```python
from build123d import *

# Parameters (mm, degrees)
SKETCH007_R           = 2.1
PAD004_DEPTH          = 1.83
CHAMFER_SIZE          = 1.6
SKETCH010_R           = 6
SKETCH010_W           = 10.4
SKETCH010_H           = 8.5
POCKET003_DEPTH       = 5
SKETCH012_R           = 3
SKETCH012_R_2         = 1.45
PAD005_DEPTH          = 4.5
SKETCH011_R           = 1.75
SKETCH011_R_2         = 3.5
SKETCH011_W           = 60.65
SKETCH011_H           = 46.16
POCKET004_DEPTH       = 7.5
CHAMFER001_SIZE       = 1
SKETCH013_W           = 70.5
SKETCH013_H           = 53
POCKET005_DEPTH       = 5
POCKET005_FACE89_R    = 1.45
PAD006_DEPTH          = 0.001
PAD006_FACE88_W       = 4.5
PAD006_FACE88_H       = 3.73839
PAD007_DEPTH          = 0.001
SKETCH014_W           = 13
SKETCH014_H           = 2.5
SKETCH014_W_2         = 8
PAD008_DEPTH          = 17
SKETCH015_R           = 1.6
POCKET006_DEPTH       = 16
PAD009_DEPTH          = 1.83
SKETCH017_R           = 1.625
POCKET007_DEPTH       = 5
SKETCH018_R           = 3
PAD010_DEPTH          = 1
SKETCH019_W           = 20
SKETCH019_H           = 10
POCKET008_DEPTH       = 1.831
POCKET008_DEPTH_BACK  = 17.001
POCKET008_FACE112_R   = 3
POCKET008_FACE112_R_2 = 1.45
PAD011_DEPTH          = 12.5
PAD011_FACE77_R       = 1.45
PAD012_DEPTH          = 12.5


with BuildPart() as part:
    # Sketch007 → Pad004 (new body)
    with BuildSketch(Plane.YZ):
        with BuildLine():
            ThreePointArc((185, 49.2), (183.857716, 51.957716), (181.1, 53.1))
            Line((-2.1, 53.1), (181.1, 53.1))
            ThreePointArc((-2.1, 53.1), (-4.857716, 51.957716), (-6, 49.2))
            Line((-6, -9), (-6, 49.2))
            ThreePointArc((-6, -9), (-4.857716, -11.757716), (-2.1, -12.9))
            Line((181.1, -12.9), (-2.1, -12.9))
            ThreePointArc((181.1, -12.9), (183.857716, -11.757716), (185, -9))
            Line((185, 49.2), (185, -9))
        make_face()
        with Locations((180.25, 49.11)):
            Circle(SKETCH007_R, mode=Mode.SUBTRACT)
        with Locations((180.25, -8.91)):
            Circle(SKETCH007_R, mode=Mode.SUBTRACT)
        with Locations((-1.25, -8.91)):
            Circle(SKETCH007_R, mode=Mode.SUBTRACT)
        with Locations((-1.25, 49.11)):
            Circle(SKETCH007_R, mode=Mode.SUBTRACT)
    extrude(amount=-PAD004_DEPTH)

    # Chamfer
    chamfer_edges = [part.edges().sort_by_distance(p)[0] for p in [
        (-1.83, 178.15, -8.91),
        (-1.83, 178.15, 49.11),
        (-1.83, -3.35, 49.11),
        (-1.83, -3.35, -8.91),
    ]]
    chamfer(chamfer_edges, length=CHAMFER_SIZE)

    # Sketch010 → Pocket003 (cut)
    with BuildSketch(Plane.YZ):
        with Locations((121.17, 7)):
            Circle(SKETCH010_R)
        with Locations((102.17, 7)):
            Circle(SKETCH010_R)
        with Locations((133.08, 5.25)):
            Rectangle(SKETCH010_W, SKETCH010_H)
        with BuildLine():
            ThreePointArc((174.5, 47.45), (172, 49.95), (169.5, 47.45))
            Line((169.5, 47.45), (169.5, -7.55))
            ThreePointArc((169.5, -7.55), (172, -10.05), (174.5, -7.55))
            Line((174.5, -7.55), (174.5, 47.45))
        make_face()
        with BuildLine():
            ThreePointArc((168.5, 47.45), (166, 49.95), (163.5, 47.45))
            Line((163.5, 47.45), (163.5, -7.55))
            ThreePointArc((163.5, -7.55), (166, -10.05), (168.5, -7.55))
            Line((168.5, -7.55), (168.5, 47.45))
        make_face()
        with BuildLine():
            ThreePointArc((162.5, 47.45), (160, 49.95), (157.5, 47.45))
            Line((157.5, 47.45), (157.5, -7.55))
            ThreePointArc((157.5, -7.55), (160, -10.05), (162.5, -7.55))
            Line((162.5, -7.55), (162.5, 47.45))
        make_face()
        with BuildLine():
            ThreePointArc((156.5, 47.45), (154, 49.95), (151.5, 47.45))
            Line((151.5, 47.45), (151.5, -7.55))
            ThreePointArc((151.5, -7.55), (154, -10.05), (156.5, -7.55))
            Line((156.5, -7.55), (156.5, 47.45))
        make_face()
        with BuildLine():
            ThreePointArc((150.5, 47.45), (148, 49.95), (145.5, 47.45))
            Line((145.5, 47.45), (145.5, -7.55))
            ThreePointArc((145.5, -7.55), (148, -10.05), (150.5, -7.55))
            Line((150.5, -7.55), (150.5, 47.45))
        make_face()
        with BuildLine():
            ThreePointArc((144.5, 47.45), (142, 49.95), (139.5, 47.45))
            Line((139.5, 47.45), (139.5, -7.55))
            ThreePointArc((139.5, -7.55), (142, -10.05), (144.5, -7.55))
            Line((144.5, -7.55), (144.5, 47.45))
        make_face()
    extrude(amount=-POCKET003_DEPTH, mode=Mode.SUBTRACT)

    # Sketch012 → Pad005 (join)
    with BuildSketch(Plane.YZ):
        with Locations((3.90349, -3.209935)):
            Circle(SKETCH012_R)
        with Locations((3.90349, -3.209935)):
            Circle(SKETCH012_R_2, mode=Mode.SUBTRACT)
        with Locations((3.90349, 41.790065)):
            Circle(SKETCH012_R)
        with Locations((3.90349, 41.790065)):
            Circle(SKETCH012_R_2, mode=Mode.SUBTRACT)
        with Locations((78.90349, 41.790065)):
            Circle(SKETCH012_R)
        with Locations((78.90349, 41.790065)):
            Circle(SKETCH012_R_2, mode=Mode.SUBTRACT)
        with Locations((120.90349, 41.790065)):
            Circle(SKETCH012_R)
        with Locations((120.90349, 41.790065)):
            Circle(SKETCH012_R_2, mode=Mode.SUBTRACT)
        with Locations((120.90349, 26.790065)):
            Circle(SKETCH012_R)
        with Locations((120.90349, 26.790065)):
            Circle(SKETCH012_R_2, mode=Mode.SUBTRACT)
        with Locations((78.90349, -3.209935)):
            Circle(SKETCH012_R)
        with Locations((78.90349, -3.209935)):
            Circle(SKETCH012_R_2, mode=Mode.SUBTRACT)
    extrude(amount=PAD005_DEPTH)

    # Sketch011 → Pocket004 (cut, symmetric)
    with BuildSketch(Plane.YZ):
        with Locations((123.990425, 34.297939)):
            Circle(SKETCH011_R)
        with Locations((95.603424, 33.973652)):
            Circle(SKETCH011_R_2)
        with Locations((44.465, 19.08)):
            Rectangle(SKETCH011_W, SKETCH011_H)
        Polygon((116.776336, 42.158814), (116.776336, 30.158814), (106.776336, 30.158814), (106.776336, 42.158814), (107.776336, 42.158814), (107.776336, 31.158814), (115.776336, 31.158814), (115.776336, 42.158814), align=None)
    extrude(amount=POCKET004_DEPTH, both=True, mode=Mode.SUBTRACT)

    # Chamfer001
    chamfer001_edges = [part.edges().sort_by_distance(p)[0] for p in [
        (-1.83, 74.79, 19.08),
        (-1.83, 44.465, 42.16),
        (-1.83, 14.14, 19.08),
        (-1.83, 44.465, -4),
    ]]
    chamfer(chamfer001_edges, length=CHAMFER001_SIZE)

    # Sketch013 → Pocket005 (cut)
    with BuildSketch(Plane.YZ):
        with Locations((41.5, 19.4)):
            Rectangle(SKETCH013_W, SKETCH013_H)
    extrude(amount=POCKET005_DEPTH, mode=Mode.SUBTRACT)

    # Pocket005 Face89 → Pad006 (add)
    with BuildSketch(Plane(origin=(4.5, 3.685812, -3.209935), x_dir=(0, -1, 0), z_dir=(1, 0, 0))):
        with BuildLine():
            Line((-2.564188, 1.869195), (-2.564188, -1.869195))
            ThreePointArc((-2.564188, -1.869195), (2.782322, 0), (-2.564188, 1.869195))
        make_face()
        with Locations((-0.217678, 0)):
            Circle(POCKET005_FACE89_R, mode=Mode.SUBTRACT)
    extrude(amount=PAD006_DEPTH)

    # Pad006 Face88 → Pad007 (add)
    with BuildSketch(Plane(origin=(2.25, 6.25, -3.209935), x_dir=(1, 0, 0), z_dir=(0, 1, 0))):
        Rectangle(PAD006_FACE88_W, PAD006_FACE88_H)
    extrude(amount=PAD007_DEPTH)

    # Sketch014 → Pad008 (join)
    with BuildSketch(Plane.YZ):
        with Locations((90.5, -6.25)):
            Rectangle(SKETCH014_W, SKETCH014_H)
        with Locations((173, -6.25)):
            Rectangle(SKETCH014_W_2, SKETCH014_H)
    extrude(amount=PAD008_DEPTH)

    # Sketch015 → Pocket006 (cut, symmetric)
    with BuildSketch(Plane.XY):
        with Locations((11.8, 173.5)):
            Circle(SKETCH015_R)
        with Locations((11.8, 89.5)):
            Circle(SKETCH015_R)
    extrude(amount=POCKET006_DEPTH, both=True, mode=Mode.SUBTRACT)

    # Sketch016 → Pad009 (join)
    with BuildSketch(Plane.YZ):
        with BuildLine():
            Line((169.016877, 10), (169.016877, -11))
            Line((169.016877, -11), (175.016877, -11))
            Line((175.016877, -11), (175.016877, 10))
            ThreePointArc((169.016877, 10), (172.016877, 7), (175.016877, 10))
        make_face()
    extrude(amount=-PAD009_DEPTH)

    # Sketch017 → Pocket007 (cut)
    with BuildSketch(Plane.YZ):
        with Locations((173.501823, 3.91)):
            Circle(SKETCH017_R)
        with Locations((89.501823, 3.91)):
            Circle(SKETCH017_R)
        with BuildLine():
            ThreePointArc((133, -10.05), (135.5, -7.55), (133, -5.05))
            Line((133, -5.05), (100, -5.05))
            ThreePointArc((100, -5.05), (97.5, -7.55), (100, -10.05))
            Line((100, -10.05), (133, -10.05))
        make_face()
    extrude(amount=-POCKET007_DEPTH, mode=Mode.SUBTRACT)

    # Sketch018 → Pad010 (join)
    with BuildSketch(Plane.YZ):
        with Locations((111.649826, 34.942547)):
            Circle(SKETCH018_R)
    extrude(amount=PAD010_DEPTH)

    # Sketch019 → Pocket008 (cut, two sides)
    with BuildSketch(Plane.YZ) as pocket008_sk:
        with Locations((116, 19.3)):
            Rectangle(SKETCH019_W, SKETCH019_H)
    extrude(amount=-POCKET008_DEPTH, mode=Mode.SUBTRACT)
    extrude(pocket008_sk.sketch, amount=POCKET008_DEPTH_BACK, mode=Mode.SUBTRACT)

    # Pocket008 Face112 → Pad011 (add)
    with BuildSketch(Plane(origin=(4.5, 120.90349, 41.790065), x_dir=(0, -1, 0), z_dir=(1, 0, 0))):
        Circle(POCKET008_FACE112_R)
        Circle(POCKET008_FACE112_R_2, mode=Mode.SUBTRACT)
    extrude(amount=PAD011_DEPTH)

    # Pad011 Face77 → Pad012 (add)
    with BuildSketch(Plane(origin=(4.5, 120.90349, 26.942319), x_dir=(0, -1, 0), z_dir=(1, 0, 0))):
        with BuildLine():
            ThreePointArc((-1.673193, 2.642319), (-2.647601, 1.563002), (-3, 0.152254))
            ThreePointArc((-3, 0.152254), (1.410748, -2.495347), (1.673193, 2.642319))
            Line((1.673193, 2.642319), (-1.673193, 2.642319))
        make_face()
        with Locations((0, 0.152254)):
            Circle(PAD011_FACE77_R, mode=Mode.SUBTRACT)
    extrude(amount=PAD012_DEPTH)


with BuildPart() as part_1:
    # Body002 placement: moved
    add(part.part.moved(Location((-0.6, 0, 0))))


solid = part_1.part
```
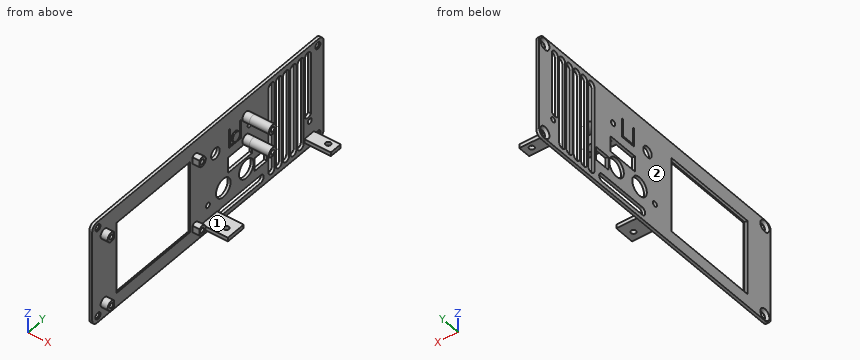
Work out the finished part from the listing and answer in its coordinate system (mm). Face numbers are marked on the shaded views. A direction names the side the tool comes from. Give positions to 0.01 mm unless a question says otherwise; leave off trailing zeros. Loops run counter-clockwise (first coordinate to the right, second up) from the corner with the lowest first, then second, coordinate; pieces in that order, holes last. Notation, with made-up numbers: (1.25, -14.75) -> (41.25, -14.75) arc R12 ccw to (41.25, 2.25) -> close; hole circle Ø1 at (47, 15). An arc over 180 degrees is marked (long way). Put each result on its own line as item: value. Start each with the question number.
Item 1: The part is cut by section A-A (y = 166). Give the vertices of the cut face in (x, z).
Item 2: The part is cut by section B-B (y = 102.17). Give the vertices of the cut face in (x, z).
Item 3: The part is cut by section D-D (z = 20.5). State how many separate pieces and enclosed holes the cut face has, then the cut area to 3 significant figures.
Item 4: Find the intervals of material crossed by L1, parallel to Z at x = -1.4, y = 121.17; L2, parallel to Z at x = -1.25, y = 110; L3, parallel to Z at x = -0.75, y = 180.25, in increasing order. Write a range as [from, to].
Item 5: The part is cut by section C-C (x = 5.75). Give the vertices of the cut face in (y, z).
Item 6: Which of the six approach directions +Z, -Z, +X, -X, +Y, -Y give full straight-line access (tool end or side, diameter ignored) to the marked faces 1 and 2?
Item 7: Each of these flat-tipped pins is pushed along its axis until it touches: P1, Ø4, axis at y = 180.25, z = 49.11, coming from the +X side; P2, Ø1.5, axis at y = 120.5, z = -3, coming from the +X side; P3, Ø2.5, axis at y = 79.5, z = -4, coming from the +X side; P4, Ø2, axis at x = 1.5, z = 41, coming from the -Y side. Where does it stop, or does it pass through?
Answers below:
1. outline: (-2.43, -12.9) -> (-0.6, -12.9) -> (-0.6, -10.05) -> (-2.43, -10.05) -> close; (-2.43, 49.95) -> (-0.6, 49.95) -> (-0.6, 53.1) -> (-2.43, 53.1) -> close
2. outline: (-2.43, -12.9) -> (-0.6, -12.9) -> (-0.6, -10.05) -> (-2.43, -10.05) -> close; (-2.43, -5.05) -> (-0.6, -5.05) -> (-0.6, 1) -> (-2.43, 1) -> close; (-2.43, 13) -> (-0.6, 13) -> (-0.6, 53.1) -> (-2.43, 53.1) -> close
3. separate pieces: 9
3. enclosed holes: 0
3. area: 146 mm2
4. L1: [-12.9, -10.05], [-5.05, 1], [13, 14.3], [24.3, 53.1]
4. L2: [-12.9, -10.05], [-5.05, 14.3], [24.3, 30.16], [31.16, 53.1]
4. L3: [-12.9, -11.01], [-6.81, 47.01], [51.21, 53.1]
5. outline: (84, -7.5) -> (97, -7.5) -> (97, -5) -> (84, -5) -> close; circle Ø6 at (120.9, 41.79); (119.23, 24.3) -> (122.58, 24.3) arc R3 ccw to (123.9, 26.79) arc R3 ccw (long way) to start; (169, -7.5) -> (177, -7.5) -> (177, -5) -> (169, -5) -> close; hole circle Ø2.9 at (120.9, 26.79); hole circle Ø2.9 at (120.9, 41.79)
6. face 1: +Z, +X, +Y
6. face 2: +Z, -Z, -X, +Y, -Y
7. P1: through
7. P2: x = -0.6
7. P3: x = 3.9
7. P4: y = 0.9
